The listing builds one solid part. Answer for the finished solid, in the listing's coordinates (mm). A direction names the side the tool comes from. Coordinates: 2 decimals unless noted, no trailing zeros. Write each loop counter-clockwise with the first axis right and the second up, starting at its lowest first coordinate (ties: lowest second). Pieces come first, ordered by that corner, then holes.
from build123d import *

# Parameters (mm, degrees)
SKETCH1_W                      = 30.121125575
SKETCH1_H                      = 11.523232915
BOSS_EXTRUDE1_DEPTH            = 4
SKETCH2_W                      = 0.023452759
SKETCH2_H                      = 13.5
CUT_EXTRUDE1_DEPTH             = 4
SKETCH3_W                      = 11.499780156
SKETCH3_H                      = 13.5
BOSS_EXTRUDE2_DEPTH            = 19
CUT_EXTRUDE2_DEPTH             = 47.721095233
DRAFT1_ANGLE                   = -45.58058215
SKETCH5_W                      = 11.499780156
SKETCH5_H                      = 0.083772182
CUT_EXTRUDE3_DEPTH             = 6.630261323
SKETCH6_W                      = 20.5
SKETCH6_H                      = 11.499780156
CUT_EXTRUDE4_DEPTH             = 7.5
BOSS_EXTRUDE3_START            = 4.500219844
BOSS_EXTRUDE3_DEPTH            = 4.500219844
SKETCH8_W                      = 8.592269897
SKETCH8_H                      = 0.01006031
CUT_EXTRUDE5_DEPTH             = 12.369738677
DRAFT2_ANGLE                   = 44.41941785
FILLET1_R                      = 2
CUT_EXTRUDE6_REACH             = 50.022
SKETCH10_W                     = 3.5
SKETCH10_H                     = 16
BOSS_EXTRUDE4_DEPTH            = 0.02681
SKETCH11_W                     = 3.5
SKETCH11_H                     = 16
BOSS_EXTRUDE5_DEPTH            = 0.02681
BOSS_EXTRUDE6_DEPTH            = 3.5
F_5_2_5_2_DIAMETER_HOLE1_D     = 5.2
F_5_2_5_2_DIAMETER_HOLE1_DEPTH = 20.621150575
F_5_0_5_DIAMETER_HOLE1_D       = 5
F_5_0_5_DIAMETER_HOLE1_DEPTH   = 4.026810169
BOSS_EXTRUDE7_START            = -4
SKETCH17_R                     = 3.5
SKETCH17_R_2                   = 2.5
BOSS_EXTRUDE7_DEPTH            = 4


with BuildPart() as part:
    # Sketch1 → Boss-Extrude1 (new body)
    with BuildSketch(Plane(origin=(16, 0, 0), x_dir=(0, -1, 0), z_dir=(-1, 0, 0))):
        with Locations((-25.560562788, 220.238163699)):
            Rectangle(SKETCH1_W, SKETCH1_H)
    extrude(amount=-BOSS_EXTRUDE1_DEPTH)

    # Sketch2 → Cut-Extrude1 (cut)
    with BuildSketch(Plane(origin=(20, 0, 0), x_dir=(0, 0, -1), z_dir=(1, 0, 0))):
        with Locations((-214.488273621, 17.25)):
            Rectangle(SKETCH2_W, SKETCH2_H)
    extrude(amount=-CUT_EXTRUDE1_DEPTH, mode=Mode.SUBTRACT)

    # Sketch3 → Boss-Extrude2 (add)
    with BuildSketch(Plane.ZY.offset(-16)):
        with Locations((220.249890078, 17.25)):
            Rectangle(SKETCH3_W, SKETCH3_H)
    extrude(amount=BOSS_EXTRUDE2_DEPTH)

    # Sketch4 → Cut-Extrude2 (cut, through all)
    with BuildSketch(Plane.XY.offset(225.999780156)):
        with BuildLine():
            Line((1, 10.5), (20, 10.5))
            Line((20, 10.5), (20, 12.5))
            Line((20, 12.5), (1, 12.5))
            ThreePointArc((1, 12.5), (2, 11.5), (1, 10.5))
        make_face()
    extrude(amount=-CUT_EXTRUDE2_DEPTH, mode=Mode.SUBTRACT)

    # Draft1
    draft1_faces = [part.faces().sort_by_distance(p)[0] for p in [
        (18, 40.621125575, 220.238163698),
    ]]
    draft(draft1_faces, Plane(origin=(20, 0, 0), x_dir=(0, 0, 1), z_dir=(1, 0, 0)), DRAFT1_ANGLE)

    # Sketch5 → Cut-Extrude3 (cut)
    with BuildSketch(Plane.ZY.offset(3)):
        with Locations((220.249890078, 23.958113909)):
            Rectangle(SKETCH5_W, SKETCH5_H)
    extrude(amount=-CUT_EXTRUDE3_DEPTH, mode=Mode.SUBTRACT)

    # Sketch6 → Cut-Extrude4 (cut)
    with BuildSketch(Plane.XZ.offset(-12.5)):
        with Locations((9.75, 220.249890078)):
            Rectangle(SKETCH6_W, SKETCH6_H)
    extrude(amount=-CUT_EXTRUDE4_DEPTH, mode=Mode.SUBTRACT)

    # Sketch7 → Boss-Extrude3 (add)
    with BuildSketch(Plane.XY.offset(225.999780156).offset(BOSS_EXTRUDE3_START)):
        with BuildLine():
            Line((-3, 10.5), (-3, 23.916227818))
            Line((-3, 23.916227818), (3.630261323, 23.916227818))
            Line((3.630261323, 23.916227818), (3.630261323, 24))
            Line((3.630261323, 24), (16, 24))
            Line((16, 24), (16, 36.539228341))
            Line((16, 36.539228341), (20, 40.621125575))
            Line((20, 40.621125575), (20, 20))
            Line((20, 20), (-0.5, 20))
            Line((-0.5, 20), (-0.5, 12.5))
            Line((-0.5, 12.5), (1, 12.5))
            ThreePointArc((1, 12.5), (2, 11.5), (1, 10.5))
            Line((1, 10.5), (-3, 10.5))
        make_face()
    extrude(amount=-BOSS_EXTRUDE3_DEPTH)

    # Sketch8 → Cut-Extrude5 (cut)
    with BuildSketch(Plane.ZY.offset(-3.630261323)):
        with Locations((226.203865052, 23.994969845)):
            Rectangle(SKETCH8_W, SKETCH8_H)
    extrude(amount=-CUT_EXTRUDE5_DEPTH, mode=Mode.SUBTRACT)

    # Draft2
    draft2_faces = [part.faces().sort_by_distance(p)[0] for p in [
        (3.630261323, 23.955573176, 222.244667153),
    ]]
    draft(draft2_faces, Plane(origin=(3.630261323, 23.916227818, 214.5), x_dir=(0, 0, 1), z_dir=(0, 1, 0)), DRAFT2_ANGLE)

    # Fillet1
    fillet1_edges = [part.edges().sort_by_distance(p)[0] for p in [
        (-3, 10.5, 222.5),
        (-3, 23.916227818, 222.5),
    ]]
    fillet(fillet1_edges, radius=FILLET1_R)

    # Sketch9 → Cut-Extrude6 (cut, up to next)
    with BuildSketch(Plane.XY.offset(214.5), mode=Mode.PRIVATE) as cut_extrude6_sk1:
        Polygon((20, 40), (20, 40.621125575), (19.391336391, 40), align=None)
    cut_extrude6_tool1 = extrude(cut_extrude6_sk1.sketch, amount=-CUT_EXTRUDE6_REACH, mode=Mode.PRIVATE) & part.part
    add(cut_extrude6_tool1.solids().sort_by_distance((19.797112, 40.207042, 214.5))[0], mode=Mode.SUBTRACT)

    # Sketch10 → Boss-Extrude4 (add)
    with BuildSketch(Plane(origin=(20.026810169, 0, 0), x_dir=(0, 0, -1), z_dir=(1, 0, 0))):
        with Locations((-216.226547241, 32)):
            Rectangle(SKETCH10_W, SKETCH10_H)
    extrude(amount=-BOSS_EXTRUDE4_DEPTH)

    # Sketch11 → Boss-Extrude5 (add)
    with BuildSketch(Plane(origin=(20.026810169, 0, 0), x_dir=(0, 0, -1), z_dir=(1, 0, 0))):
        with Locations((-228.683158875, 32)):
            Rectangle(SKETCH11_W, SKETCH11_H)
    extrude(amount=-BOSS_EXTRUDE5_DEPTH)

    # Sketch12 → Boss-Extrude6 (add)
    with BuildSketch(Plane(origin=(0, 0, 214.476547241), x_dir=(-1, 0, 0), z_dir=(0, 0, -1))):
        Polygon((-16, 24), (-3.71235274, 24), (-16, 36.539228341), align=None)
    extrude(amount=-BOSS_EXTRUDE6_DEPTH)

    # Ø5.2 (5.2) Diameter Hole1
    with Locations(Plane(origin=(0, 20, 0), x_dir=(-1, 0, 0), z_dir=(0, -1, 0))):
        with Locations((-10, -222.5)):
            Hole(F_5_2_5_2_DIAMETER_HOLE1_D / 2, depth=F_5_2_5_2_DIAMETER_HOLE1_DEPTH)

    # Ø5.0 (5) Diameter Hole1
    with Locations(Plane.ZY.offset(-16)):
        with Locations((222.5, 36.5)):
            Hole(F_5_0_5_DIAMETER_HOLE1_D / 2, depth=F_5_0_5_DIAMETER_HOLE1_DEPTH)

    # Sketch17 → Boss-Extrude7 (add)
    with BuildSketch(Plane.ZY.offset(-16).offset(BOSS_EXTRUDE7_START)):
        with Locations((222.5, 36.5)):
            Circle(SKETCH17_R)
        with Locations((222.5, 36.5)):
            Circle(SKETCH17_R_2, mode=Mode.SUBTRACT)
    extrude(amount=BOSS_EXTRUDE7_DEPTH)


solid = part.part
1. A tool of negligible diameter and unlimited length cuts with its end or side. For faces 5 (the cylindrical face through (17.3, 40, 222.6)), 6 (the flat face through (-0.5, 16, 223)), 7 (the flat face through (9.8, 24, 219.5)), 8 (the flat face through (1, 23.916, 223)), 9 (the flat face through (20.027, 32, 216)), from which of +Z, -Z, +X, -X, +Y, -Y can it reach the whole face along a straight path? Write none if from no direction.
Results found:
face 5: -X, +Y
face 6: +Z, -Z, +X
face 7: +Z, -X, +Y
face 8: +Z, -Z, -X, +Y
face 9: +Z, -Z, +X, +Y, -Y
2. Find the intervals of material crossed by L1, parallel to Z at x = 18.35, y = 36.5; L2, parallel to Z at x = 10, y = 22.9; L3, parallel to Y at x = 19, z = 222.5, in increasing order.
Results found:
L1: z = 214.48 to 220, 225 to 230.5
L2: z = 214.5 to 219.9, 225.1 to 230.5
L3: y = 20 to 34, 39 to 40
3. For a pull along X with two mould halves and no side action, classify faces 1 (the cylindrical face through (9.662, 22.028, 219.922)), 2 (the flat face through (-3, 17, 223)), 3 (the cylindrical face through (2, 11.5, 222.6)), 4 (the flat face through (10, 23.99, 226)) as pulls with the +X half, pulls with the -X half, needs draft (parallel to the pull), parting line crosses it, or undercut.
Results found:
face 1: undercut
face 2: pulls with the -X half
face 3: pulls with the +X half
face 4: needs draft
4. Section A-A on z = 222.5 is taken. Give the vertices of the cut face in (x, y).
Results found:
outline: (-3, 12.5) arc R2 ccw to (-1, 10.5) - (1, 10.5) arc R1 ccw to (1, 12.5) - (-0.5, 12.5) - (-0.5, 20) - (7.4, 20) - (7.4, 23.99) - (3.7, 23.99) - (3.63, 23.92) - (-1, 23.92) arc R2 ccw to (-3, 21.92) - close; (12.6, 20) - (20, 20) - (20, 34) - (16, 34) - (16, 23.99) - (12.6, 23.99) - close; (16, 39) - (20, 39) - (20, 40.62) - (19.39, 40) - (16, 40) - close
5. Flat-ended cylindrical pins translate along their axes: P1, Ø1.2, axis at x = 9, z = 219.5, coming from the +Y side; P2, Ø6, axis at x = 10, z = 222.5, coming from the -Y side; P3, Ø3, axis at x = 4.5, z = 218, coming from the +Y side; P4, Ø7, axis at x = 7, y = 15.5, coming from the -Z side. Find the tip coordinate at first contact, or state that the pin passes through.
Results found:
P1: stops at y = 24
P2: stops at y = 20
P3: stops at y = 26.33
P4: passes through
